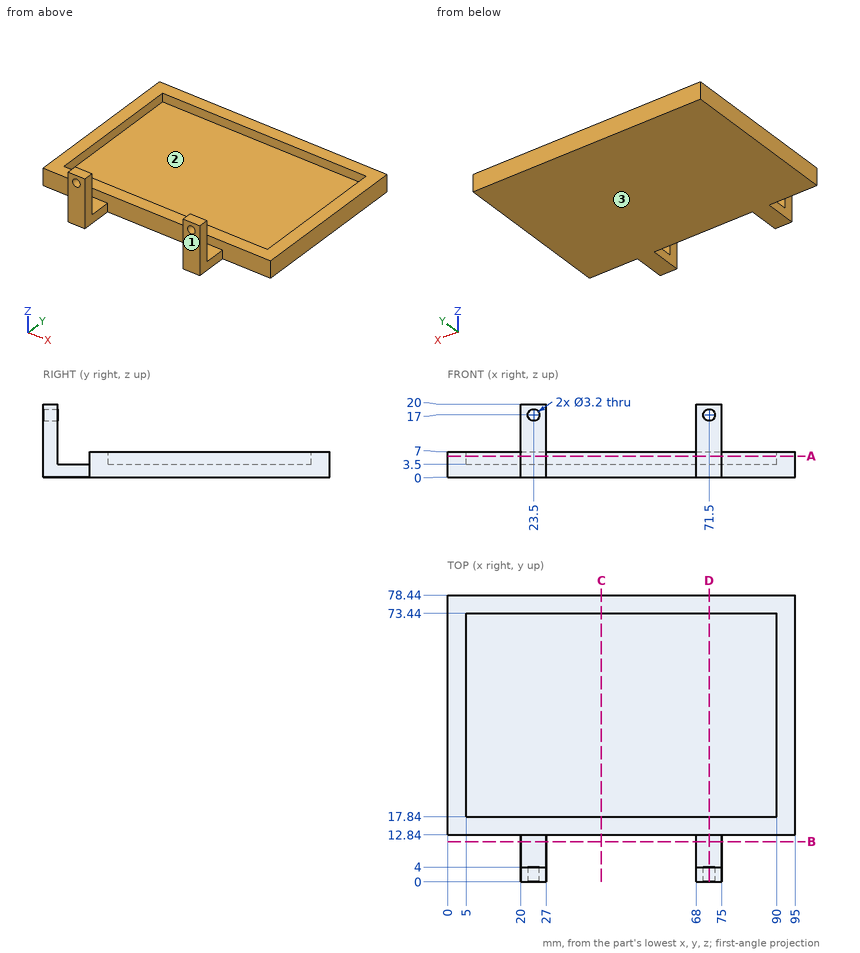
The drawing under review shows one solid part. Ordinate dimensions are in mm from its lowest x, y, z. Give positions to 0.01 mm unless a question says otherwise; leave off trailing zeros. Write each loop counter-clockwise with the first axis right and the second up, starting at its lowest first coordinate (ties: lowest second). Pieces come first, ordered by that corner, then holes. Notation, with made-up numbers: (47.25, 43.25) -> (78.25, 43.25) arc R23 ccw to (78.25, 61.25) -> close; hole circle Ø5 at (37.25, 64). An arc over 180 degrees is marked (long way). Use CSV: the item, a comma, the result in double quotes.
Q1. Take a section at D-D, the plane x = 71.5. Write out the cut boundary in (y, z), then the cut area to 3 significant figures.
Conclusion:
outline,"(0, 0) -> (78.44, 0) -> (78.44, 7) -> (73.44, 7) -> (73.44, 3.5) -> (17.84, 3.5) -> (17.84, 7) -> (12.84, 7) -> (12.84, 3.5) -> (4, 3.5) -> (4, 15.4) -> (0, 15.4) -> close; (0, 18.6) -> (4, 18.6) -> (4, 20) -> (0, 20) -> close"
area,"363 mm2"
Q2. Take a section at A-A, the plane z = 5.75. Write out the cut boundary in (x, y), then the cut area to 3 significant figures.
Conclusion:
outline,"(0, 12.84) -> (95, 12.84) -> (95, 78.44) -> (0, 78.44) -> close; (20, 0) -> (27, 0) -> (27, 4) -> (20, 4) -> close; (68, 0) -> (75, 0) -> (75, 4) -> (68, 4) -> close; hole (5, 17.84) -> (90, 17.84) -> (90, 73.44) -> (5, 73.44) -> close"
area,"1,560 mm2"
Q3. Mouldability with a two-part tool opening along Y and no side actions: class the marked faces 1, 2 and 3 as pulls with the +Y half, pulls with the -Y half, needs draft (parallel to the pull), parting line crosses it, or undercut.
Conclusion:
face 1,"pulls with the -Y half"
face 2,"undercut"
face 3,"needs draft"
Q4. To check wall thickness, follow probe 1 along Z at (x, y) = (23.5, 2.7); probe 2 along X at (y, z) = (55, 4.5); probe 3 along Y at (x, z) = (28.5, 5). State the ranges of each line that lie inside material, in increasing order. Write a range as [from, to].
Conclusion:
probe 1,"[0, 15.4], [18.6, 20]"
probe 2,"[0, 5], [90, 95]"
probe 3,"[12.84, 17.84], [73.44, 78.44]"
Q5. Take a section at C-C, the plane x = 42. Write out the cut boundary in (y, z).
Conclusion:
outline,"(12.84, 0) -> (78.44, 0) -> (78.44, 7) -> (73.44, 7) -> (73.44, 3.5) -> (17.84, 3.5) -> (17.84, 7) -> (12.84, 7) -> close"
Q6. For P1, Ø1.9, axis at x = 23.5, z = 17, coming from the +Y side; P2, Ø2, axis at x = 66, y = 67.5, coming from the +Z side; P3, Ø1.5, axis at x = 58, z = 7, coming from the -Y side; P4, Ø4, axis at y = 5, z = 13.5, coming from the +X side, all flat-tipped, find the tip position at first contact; note any pin that passes through.
Conclusion:
P1,"through"
P2,"z = 3.5"
P3,"y = 12.84"
P4,"x = 75"
Q7. Take a section at B-B, the plane y = 11. Write out the cut boundary in (x, z).
Conclusion:
outline,"(20, 0) -> (27, 0) -> (27, 3.5) -> (20, 3.5) -> close; (68, 0) -> (75, 0) -> (75, 3.5) -> (68, 3.5) -> close"
